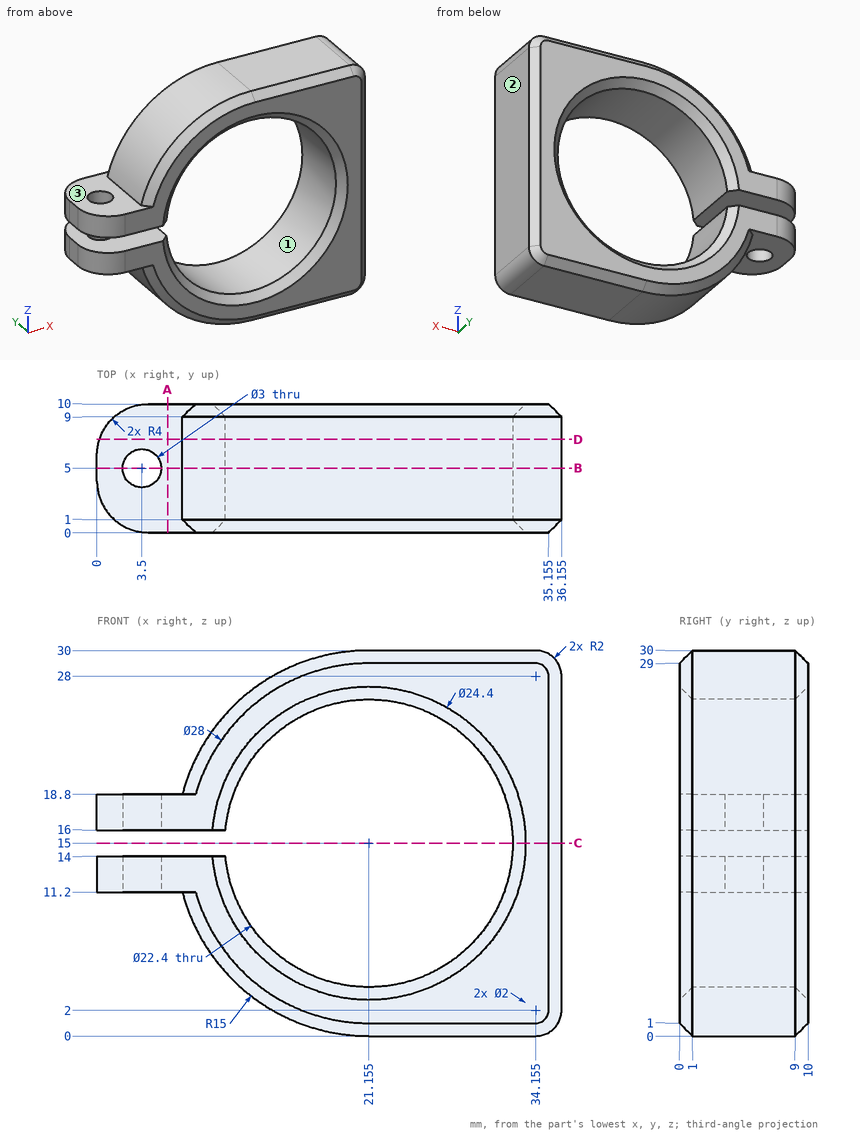
Design review of the part shown in the three views and the two pictorial views. Dimensions are in mm from the part's minimum x, y and z. Round coordinates to 2 decimals unless told otherwise and drop trailing zeros. Loops run counter-clockwise (first coordinate to the right, second up) from the corner with the lowest first, then second, coordinate; pieces in that order, holes last.
Q1. Mouldability with a two-part tool opening along Z and no side actions: class the marked faces 1, 2 and 3 as +Z half, -Z half, draft (parallel to the pull), parting line (faces both ways), or undercut.
Result sheet:
face 1: undercut
face 2: draft
face 3: +Z half
Q2. Add section A-A on x = 5.5. Write out the cut boundary in (y, z).
Result sheet:
outline: (0, 11.2) - (10, 11.2) - (10, 14) - (0, 14) - close; (0, 16) - (10, 16) - (10, 18.8) - (0, 18.8) - close
Q3. Add section B-B on y = 5. Write out the cut boundary in (x, z) (1 decimal).
Result sheet:
outline: (0, 11.2) - (2, 11.2) - (2, 14) - (0, 14) - close; (0, 16) - (2, 16) - (2, 18.8) - (0, 18.8) - close; (5, 11.2) - (6.6, 11.2) arc R15 ccw to (21.2, 0) - (34.2, 0) arc R2 ccw to (36.2, 2) - (36.2, 28) arc R2 ccw to (34.2, 30) - (21.2, 30) arc R15 ccw to (6.6, 18.8) - (5, 18.8) - (5, 16) - (10, 16) arc R11.2 cw (long way) to (10, 14) - (5, 14) - close
Q4. Add section C-C on z = 15. Write out the cut boundary in (x, y) (1 decimal), plus the area to 3 significant figures.
Result sheet:
outline: (32.4, 1) - (33.4, 0) - (35.2, 0) - (36.2, 1) - (36.2, 9) - (35.2, 10) - (33.4, 10) - (32.4, 9) - close
area: 36.0 mm2
Q5. Insertion check: pin 1 Ø5 at (x, y) = (3, 4.5) entering from +Z; pin 2 Ø1.5 at (x, y) = (11, 1.5) entering from -Z (1 decimal); pin 3 Ø6 at (x, y) = (5.5, 5.5) entering from +Z. Each pin has a flat end and moves straight along its axis. Give the tip position at first contact, or say it passes through.
Result sheet:
pin 1: stops at z = 18.8
pin 2: stops at z = 3.3
pin 3: stops at z = 23.05
Q6. To check wall thickness, follow line 1 along X through (y, z) = (5, 13) (1 decimal); line 2 along Z through (x, y) = (3, 8.75); line 3 along X through (y, z) = (5.25, 11.25) (1 decimal). State the ranges of each line that lie inside material, in increasing order.
Result sheet:
line 1: x = 0 to 2, 5 to 10.1, 32.2 to 36.2
line 2: z = 11.2 to 14, 16 to 18.8
line 3: x = 0 to 2, 5 to 10.6, 31.7 to 36.2
Q7. Add section D-D on y = 7.25. Write out the cut boundary in (x, z) (1 decimal).
Result sheet:
outline: (0.2, 11.2) - (6.6, 11.2) arc R15 ccw to (21.2, 0) - (34.2, 0) arc R2 ccw to (36.2, 2) - (36.2, 28) arc R2 ccw to (34.2, 30) - (21.2, 30) arc R15 ccw to (6.6, 18.8) - (0.2, 18.8) - (0.2, 16) - (10, 16) arc R11.2 cw (long way) to (10, 14) - (0.2, 14) - close
